Here's how the part is built. I have some questions about the finished solid (model axes, mm). A direction names the side the tool comes from. Give positions to 0.01 mm unless a question says otherwise; leave off trailing zeros. Loops run counter-clockwise (first coordinate to the right, second up) from the corner with the lowest first, then second, coordinate; pieces in that order, holes last. Notation, with made-up numbers: (41, 25.5) - (45, 25.5) arc R10 cw to (45, 43.5) - close; hole circle Ø5 at (-35.5, 46.5). An arc over 180 degrees is marked (long way). Put each result on its own line as item: value. Start each with the question number.
from build123d import *

# Parameters (mm, degrees)
SKETCH_W        = 10
SKETCH_H        = 17
PAD_DEPTH       = 23
SKETCH001_W     = 9
SKETCH001_H     = 8
POCKET_DEPTH    = 20
SKETCH002_R     = 2
POCKET001_DEPTH = 30
SKETCH003_W     = 8
SKETCH003_H     = 1.6
POCKET002_DEPTH = 8
SKETCH004_R     = 0.7
PAD001_DEPTH    = 8
SKETCH005_W     = 6
SKETCH005_H     = 9
POCKET003_DEPTH = 10


with BuildPart() as part:
    # Sketch → Pad (new body)
    with BuildSketch(Plane.ZY):
        with Locations((-44.312478, 27.275098)):
            Rectangle(SKETCH_W, SKETCH_H)
    extrude(amount=PAD_DEPTH)

    # Sketch001 → Pocket (cut)
    with BuildSketch(Plane(origin=(0, 0, -39.312478), x_dir=(0, 1, 0), z_dir=(0, 0, 1))):
        with Locations((31.275098, 4)):
            Rectangle(SKETCH001_W, SKETCH001_H)
    extrude(amount=-POCKET_DEPTH, mode=Mode.SUBTRACT)

    # Sketch002 → Pocket001 (cut)
    with BuildSketch(Plane(origin=(-8, 0, 0), x_dir=(0, 0, 1), z_dir=(1, 0, 0))):
        with Locations((-43.312478, -31.775098)):
            Circle(SKETCH002_R)
    extrude(amount=-POCKET001_DEPTH, mode=Mode.SUBTRACT)

    # Sketch003 → Pocket002 (cut)
    with BuildSketch(Plane(origin=(0, 18.775098, 0), x_dir=(0, 0, 1), z_dir=(0, -1, 0))):
        with Locations((-43.312478, 4.2)):
            Rectangle(SKETCH003_W, SKETCH003_H)
    extrude(amount=-POCKET002_DEPTH, mode=Mode.SUBTRACT)

    # Sketch004 → Pad001 (new body)
    with BuildSketch(Plane(origin=(0, 0, -39.312478), x_dir=(0, 1, 0), z_dir=(0, 0, 1))):
        with Locations((19.775098, 3.4)):
            Circle(SKETCH004_R)
        with Locations((21.775098, 3.4)):
            Circle(SKETCH004_R)
        with Locations((23.775098, 3.4)):
            Circle(SKETCH004_R)
        with Locations((25.775098, 3.4)):
            Circle(SKETCH004_R)
    extrude(amount=-PAD001_DEPTH)

    # Sketch005 → Pocket003 (cut)
    with BuildSketch(Plane(origin=(0, 0, -39.312478), x_dir=(0, 1, 0), z_dir=(0, 0, 1))):
        with Locations((24.775098, 15.5)):
            Rectangle(SKETCH005_W, SKETCH005_H)
    extrude(amount=-POCKET003_DEPTH, mode=Mode.SUBTRACT)


solid = part.part
1) Which directions (+Z, -Z, +X, -X, +Y, -Y) give clear straight access to the entire face, cutting with the end or side of a thin tool? Please do faces 1 (the flat face through (-11, 25, -44)), 2 (the flat face through (-3, 26.775, -44)), 3 (the flat face through (-5, 23, -43)), 4 (the cylindrical face through (-4.1, 23.8, -43.3)).
2) Suppose I cut it at A-A on z = -46. Please give me the cut outline in (x, y), plus the area to 3 significant figures.
3) Thinking about a two-plate mould opening in X: for faces 5 (the cylindrical face through (-4.1, 25.8, -43.3)), 6 (the flat face through (-23, 27, -44)), 7 (the flat face through (-2, 23, -39.312)), which applies, pulls with the +X half, pulls with the -X half, needs draft (parallel to the pull), parting line crosses it, or undercut?
4) Suppose I cut it at D-D on z = -47.75. Please give me the cut outline in (x, y).
5) I need wall thicknesses on line 1 (X direction, y = 25.75, z = -42); line 2 (Y direction, x = -15, z = -42); line 3 (Y direction, x = -12.75, z = -42.5). Which ranges of each line are inside material? Lowest first, please.
6) I'm going to push a flat-ended pin straight in: P1, Ø2.5, axis at x = -6, z = -44.5, coming from the +Y side. Where does the tip first touch, or does it pass through?
7) Suppose I cut it at C-C on x = -13.25. Please give me the cut outline in (y, z), plus the area to 3 significant figures.
8) Suppose I cut it at B-B on z = -44.5. Please give me the cut outline in (x, y).
Ans:
1. face 1: +Z, -Z
1. face 2: +Z, -Z, +X, +Y
1. face 3: +Z, +Y, -Y
1. face 4: +Z
2. outline: (-23, 18.78) - (-5, 18.78) - (-5, 26.78) - (-8, 26.78) - (-8, 35.78) - (-23, 35.78) - close; (-3.4, 18.78) - (0, 18.78) - (0, 26.78) - (-3.4, 26.78) - (-3.4, 26.48) arc R0.7 ccw to (-3.4, 25.08) - (-3.4, 24.48) arc R0.7 ccw to (-3.4, 23.08) - (-3.4, 22.48) arc R0.7 ccw to (-3.4, 21.08) - (-3.4, 20.48) arc R0.7 ccw to (-3.4, 19.08) - close; hole (-20, 21.78) - (-11, 21.78) - (-11, 27.78) - (-20, 27.78) - close
2. area: 255 mm²
3. face 5: undercut
3. face 6: pulls with the -X half
3. face 7: needs draft
4. outline: (-23, 18.78) - (0, 18.78) - (0, 26.78) - (-8, 26.78) - (-8, 35.78) - (-23, 35.78) - close; hole (-20, 21.78) - (-11, 21.78) - (-11, 27.78) - (-20, 27.78) - close
5. line 1: x = -23 to -20, -11 to -5, -4.1 to 0
5. line 2: y = 18.78 to 21.78, 27.78 to 30.27, 33.28 to 35.78
5. line 3: y = 18.78 to 21.78, 27.78 to 29.95, 33.6 to 35.78
6. P1: stops at y = 26.78
7. outline: (18.78, -49.31) - (21.78, -49.31) - (21.78, -39.31) - (18.78, -39.31) - close; (27.78, -49.31) - (35.78, -49.31) - (35.78, -39.31) - (27.78, -39.31) - close; hole circle Ø4 at (31.78, -43.31)
7. area: 97.4 mm²
8. outline: (-23, 18.78) - (-5, 18.78) - (-5, 26.78) - (-8, 26.78) - (-8, 30.17) - (-23, 30.17) - close; (-23, 33.38) - (-8, 33.38) - (-8, 35.78) - (-23, 35.78) - close; (-3.4, 18.78) - (0, 18.78) - (0, 26.78) - (-3.4, 26.78) - (-3.4, 26.48) arc R0.7 ccw to (-3.4, 25.08) - (-3.4, 24.48) arc R0.7 ccw to (-3.4, 23.08) - (-3.4, 22.48) arc R0.7 ccw to (-3.4, 21.08) - (-3.4, 20.48) arc R0.7 ccw to (-3.4, 19.08) - close; hole (-20, 21.78) - (-11, 21.78) - (-11, 27.78) - (-20, 27.78) - close
